Input: part model. Units: mm. Frame: model coordinates. Face numbers are marked on the shaded views. A direction names the side the tool comes from. Round coordinates to 2 decimals unless told otherwise and drop trailing zeros. Loops run counter-clockwise (first coordinate to the right, second up) from the corner with the lowest first, then second, coordinate; pieces in that order, holes last. Notation, with made-up numbers: (88.5, -3) - (135.5, -3) arc R25 cw to (135.5, 25) - close; hole circle Ø4 at (26, 4). An arc over 180 degrees is marked (long way). Write each question's results on one line, items separated by ' | '.
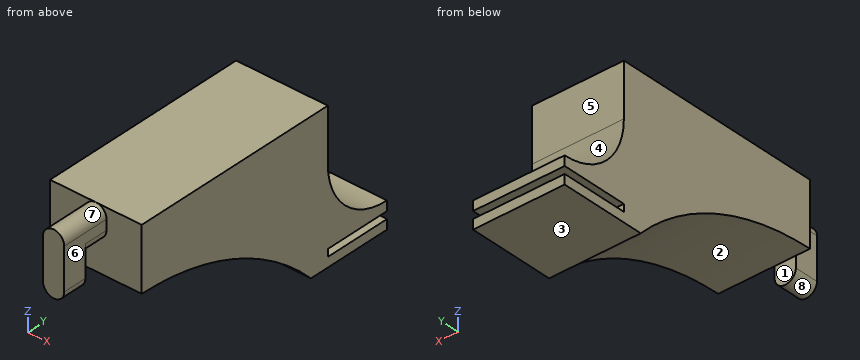
from build123d import *

# Parameters (mm, degrees)
SKETCH_W     = 19
SKETCH_H     = 18
PAD_DEPTH    = 2
SKETCH001_W  = 19
SKETCH001_H  = 4
PAD001_DEPTH = 3.5
SKETCH002_W  = 19
SKETCH002_H  = 2
PAD002_DEPTH = 14
SKETCH003_W  = 19
SKETCH003_H  = 4
PAD003_DEPTH = 14
PAD004_DEPTH = 19
PAD005_DEPTH = 19
PAD006_DEPTH = 5
PAD007_DEPTH = 5


with BuildPart() as part:
    # Sketch → Pad (new body)
    with BuildSketch(Plane.XY):
        with Locations((0, -1)):
            Rectangle(SKETCH_W, SKETCH_H)
    extrude(amount=PAD_DEPTH)

    # Sketch001 (on Face6 of Pad) → Pad001 (join)
    with BuildSketch(Plane.XY.offset(2)):
        with Locations((0, -8)):
            Rectangle(SKETCH001_W, SKETCH001_H)
    extrude(amount=PAD001_DEPTH)

    # Sketch002 (on Face4 of Pad001) → Pad002 (join)
    with BuildSketch(Plane(origin=(0, -6, 0), x_dir=(-1, 0, 0), z_dir=(0, 1, 0))):
        with Locations((0, 4.5)):
            Rectangle(SKETCH002_W, SKETCH002_H)
    extrude(amount=PAD002_DEPTH)

    # Sketch003 (on Face10 of Pad002) → Pad003 (join)
    with BuildSketch(Plane.XY.offset(5.5)):
        with Locations((0, -8)):
            Rectangle(SKETCH003_W, SKETCH003_H)
    extrude(amount=PAD003_DEPTH)

    # Sketch004 (on Face11 of Pad003) → Pad004 (join)
    with BuildSketch(Plane(origin=(-9.5, 0, 0), x_dir=(0, -1, 0), z_dir=(-1, 0, 0))):
        with BuildLine():
            Line((-8, 5.5), (6, 5.5))
            Line((6, 19.5), (6, 5.5))
            ThreePointArc((-8, 5.5), (1.899495, 9.600505), (6, 19.5))
        make_face()
    extrude(amount=-PAD004_DEPTH)

    # Sketch005 (on Face11 of Pad004) → Pad005 (join)
    with BuildSketch(Plane(origin=(-9.5, 0, 0), x_dir=(0, -1, 0), z_dir=(-1, 0, 0))):
        with BuildLine():
            Line((10, 30.5), (6, 30.5))
            Line((6, 30.5), (6, 19.5))
            Line((6, 19.5), (10, 19.5))
            Line((10, 19.5), (10, 0))
            ThreePointArc((50, 17.5), (28.169689, 12.933569), (10, 0))
            Line((50, 17.5), (50, 30.5))
            Line((50, 30.5), (10, 30.5))
        make_face()
    extrude(amount=-PAD005_DEPTH)

    # Sketch006 (on Face10 of Pad005) → Pad006 (join)
    with BuildSketch(Plane.XZ.offset(50)):
        with BuildLine():
            ThreePointArc((-2.2, 26.2), (0, 24), (2.2, 26.2))
            Line((2.2, 26.2), (2.2, 28.3))
            ThreePointArc((2.2, 28.3), (0, 30.5), (-2.2, 28.3))
            Line((-2.2, 26.2), (-2.2, 28.3))
        make_face()
    extrude(amount=PAD006_DEPTH)

    # Sketch007 (on Face18 of Pad006) → Pad007 (join)
    with BuildSketch(Plane.XZ.offset(55)):
        with BuildLine():
            ThreePointArc((2.2, 28.3), (0, 30.5), (-2.2, 28.3))
            Line((-2.2, 28.3), (-2.2, 19.7))
            ThreePointArc((-2.2, 19.7), (0, 17.5), (2.2, 19.7))
            Line((2.2, 28.3), (2.2, 19.7))
        make_face()
    extrude(amount=PAD007_DEPTH)


solid = part.part
1. Set-up query: the marked faces 5, 6, 7 and 8. Return all of +Z, -Z, +X, -X, +Y, -Y with unobstructed straight access to the full face (end or side cutting, diameter ignored); none if empty.
Answer:
face 5: +Z, +X, -X, +Y | face 6: +Z, -Z, +X, -Y | face 7: +Z, -Y | face 8: -Z, -Y
2. Section query C-C, the plane z = 9. Output: boundary loops of the cut face in (x, y).
Answer:
outline: (-9.5, -20.78) - (9.5, -20.78) - (9.5, -1.26) - (-9.5, -1.26) - close
3. Line query: line 1 (Y direction, x = 5.5, z = 21.5); line 2 (Z direction, x = 2.25, y = 4); line 3 (Z direction, x = 6.75, y = 3). Output: solid intervals per line, ascending. Write a range as [from, to].
Answer:
line 1: [-50, -6] | line 2: [0, 2], [3.5, 6.08] | line 3: [0, 2], [3.5, 6.42]
4. Section query D-D, the plane y = -52.5. Output: boundary loops of the cut face in (x, z), plus the area to 3 significant figures.
Answer:
outline: (-2.2, 26.2) arc R2.2 ccw to (2.2, 26.2) - (2.2, 28.3) arc R2.2 ccw to (-2.2, 28.3) - close | area: 24.4 mm^2
5. Mould query, pull axis Y, two halves, no side actions, for the marked faces 1, 2, 3 and 4. Classes: pulls with the +Y half, pulls with the -Y half, needs draft (parallel to the pull), parting line crosses it, or undercut.
Answer:
face 1: undercut | face 2: pulls with the -Y half | face 3: needs draft | face 4: pulls with the +Y half
6. Section query A-A, the plane y = 2. Output: boundary loops of the cut face in (x, z).
Answer:
outline: (-9.5, 0) - (9.5, 0) - (9.5, 2) - (-9.5, 2) - close; (-9.5, 3.5) - (9.5, 3.5) - (9.5, 6.85) - (-9.5, 6.85) - close
7. Contact query for flat-ended pins moving along their axis: pin 1 (5.5 mm diameter, centred on x = 2.5, z = 27, fed in from +Y); pin 2 (2 mm diameter, centred on x = -3, y = -44, fed in from -Z); pin 3 (4 mm diameter, centred on x = -1, z = 7, fed in from -Y). Output: stop coordinate, or through.
Answer:
pin 1: y = -6 | pin 2: z = 17.05 | pin 3: y = -20.78
8. Section query B-B, the plane x = -3.5. Output: boundary loops of the cut face in (y, z).
Answer:
outline: (-50, 17.5) arc R54.46 cw to (-10, 0) - (8, 0) - (8, 2) - (-6, 2) - (-6, 3.5) - (8, 3.5) - (8, 5.5) arc R14 cw to (-6, 19.5) - (-6, 30.5) - (-50, 30.5) - close
